from build123d import *

# Parameters (mm, degrees)
BOSS_EXTRUDE1_DEPTH             = 152.4
FILLET1_R                       = 3.175
F_3_4_0_75_DIAMETER_HOLE1_D     = 19.05
F_3_4_0_75_DIAMETER_HOLE1_DEPTH = 6.35


with BuildPart() as part:
    # Sketch1 → Boss-Extrude1 (new body)
    with BuildSketch(Plane(origin=(0, 0, 0), x_dir=(1, 0, 0), z_dir=(0, 1, 0))):
        Polygon((0, 0), (0, 50.8), (6.35, 50.8), (6.35, 6.35), (50.8, 6.35), (50.8, 0), align=None)
    extrude(amount=BOSS_EXTRUDE1_DEPTH)

    # Fillet1
    fillet1_edges = [part.edges().sort_by_distance(p)[0] for p in [
        (6.35, 76.2, -6.35),
    ]]
    fillet(fillet1_edges, radius=FILLET1_R)

    # 3/4 (0.75) Diameter Hole1
    with Locations(Plane.ZY):
        with Locations((-25.4, 31.75)):
            Hole(F_3_4_0_75_DIAMETER_HOLE1_D / 2, depth=F_3_4_0_75_DIAMETER_HOLE1_DEPTH)


solid = part.part
Read the model definition and answer for the solid it produces. Units are mm, in the model's axes. A direction names the side the tool comes from. Coordinates: 2 decimals unless noted, no trailing zeros. Order: outer loops, then holes, each group sorted by start corner. A loop starts at its lowest first (then second) coordinate and runs counter-clockwise, first axis right, second up. Notation, with made-up numbers: M 15.25,36 L 33.25,36 A27 cw 33.25,71 Z; hole C 37,27.5 d9. An arc over 180 degrees is marked long. Put each result on its own line as item: value. Start each with the question number.
Item 1: Section C-C, the plane y = 115.5 is taken. Determine the outline of the cut face in (x, z) (3 decimals).
Item 2: Section D-D, the plane z = -39.5 is taken. Determine the outline of the cut face in (x, y).
Item 3: Section B-B, the plane y = 31.75 is taken. Determine the outline of the cut face in (x, z) (3 decimals), plus the area to 3 significant figures.
Item 4: Given pin 1 Ø5 at (y, z) = (90.5, -28.5) entering from +X; pin 2 Ø3 at (x, y) = (11.5, 76) entering from -Z, each flat-ended and moving along its own axis, determine where each tip first touches the part or whether it passes through.
Item 5: For faces 5 (the face through (6.35, 75, -30)), 6 (the face through (0, 75, -25)), determine the directions among +Z, -Z, +X, -X, +Y, -Y from which every point of the face is accessible in a straight line to the end or side of a thin tool.
Item 6: Section A-A, the plane z = -25.4 is taken. Determine the outline of the cut face in (x, y) (3 decimals), plus the area to 3 significant figures.
Item 7: The mould has two halves that part along Y. Classify faces 1 (the face through (3.22, 22.45, -23.34)), 2 (the face through (50.8, 75, -3)), 3 (the face through (16, 152.4, -5)), 4 (the face through (16, 0, -5)): +Y half, -Y half, draft (parallel to the pull), parting line (faces both ways), or undercut.
Item 8: Consider probe 1 along Y at (x, z) = (4, -25); probe 2 along X at (y, z) = (96.5, -44.5); probe 3 along Z at (x, y) = (2, 31). Determine where each line is inside the solid, lowest interval first. Write a range as [from, to].
Computed:
1. outline: M 0,-50.8 L 6.35,-50.8 L 6.35,-9.525 A3.175 cw 9.525,-6.35 L 50.8,-6.35 L 50.8,0 L 0,0 Z
2. outline: M 0,0 L 6.35,0 L 6.35,152.4 L 0,152.4 Z
3. outline: M 0,-50.8 L 6.35,-50.8 L 6.35,-34.925 L 0,-34.925 Z; M 0,-15.875 L 6.35,-15.875 L 6.35,-9.525 A3.175 cw 9.525,-6.35 L 50.8,-6.35 L 50.8,0 L 0,0 Z
3. area: 486 mm2
4. pin 1: stops at x = 6.35
4. pin 2: stops at z = -6.35
5. face 5: -Z, +X, +Y, -Y
5. face 6: +Z, -Z, -X, +Y, -Y
6. outline: M 0,0 L 6.35,0 L 6.35,22.225 L 0,22.225 Z; M 0,41.275 L 6.35,41.275 L 6.35,152.4 L 0,152.4 Z
6. area: 847 mm2
7. face 1: undercut
7. face 2: draft
7. face 3: +Y half
7. face 4: -Y half
8. probe 1: y = [0, 22.23], [41.27, 152.4]
8. probe 2: x = [0, 6.35]
8. probe 3: z = [-50.8, -34.9], [-15.9, 0]
